The listing builds one solid part. Answer for the finished solid, in the listing's coordinates (mm). A direction names the side the tool comes from. Coordinates: 2 decimals unless noted, no trailing zeros. Order: outer loops, then holes, each group sorted by start corner. A loop starts at its lowest first (then second) coordinate and runs counter-clockwise, first axis right, second up. Notation, with made-up numbers: (42.5, 20) - (58.5, 20) arc R26 cw to (58.5, 49) - close; hole circle Ø4 at (-13, -4). An arc over 180 degrees is marked (long way). Use a Markdown table: item, result. Add a question column.
Item 1: The mould has two halves that part along X. Classify faces 1 (the flat face through (5, 38, 1)), 2 (the flat face through (-155, 38, 1)), 3 (the cylindrical face through (-43.2, -41, 130.3)): released by +X, released by -X, zero draft, split by the parting line, or undercut.
Item 2: For faces 4 (the cylindrical face through (-73.88, 1.32, 29.97)), 5 (the cylindrical face through (-149.93, 85.907, -19.077)), 6 (the flat face through (-5, 69, -69)), 7 (the flat face through (-25, -1, -137)), determine the directions among +Z, -Z, +X, -X, +Y, -Y from which every point of the face is accessible in a straight line to the end or side of a thin tool.
Item 3: Find the intervals of material crossed by line 1 along Y through (x, z) = (-34.5, 0); line 2 along X through (y, z) = (-25, -141.5); line 3 along X through (y, z) = (109.5, 16.5), in increasing order.
Item 4: The part is cut by section C-C, the plane x = -117. Give the vertices of the cut face in (y, z), then the cut area to 3 significant figures.
Item 5: Flat-ended cylindrical pins translate along their axes: P1, Ø3, axis at x = -120, y = -101.5, coming from the -Z side; P2, Ø3, axis at y = 83, z = -92.5, coming from the +X side; P3, Ø5, axis at x = -104.5, y = 104.5, coming from the -Z side. Find the tip coordinate at first contact, or state that the pin passes through.
from build123d import *

# Parameters (mm, degrees)
SKETCH1_W          = 10
SKETCH1_H          = 88
SKETCH1_W_2        = 37
SKETCH1_H_2        = 136.59637726
SKETCH2_R          = 30
CUT_EXTRUDE1_DEPTH = 500


with BuildPart() as part:
    # Sketch1 → Revolve9 (revolve)
    with BuildSketch(Plane.XY, mode=Mode.PRIVATE) as revolve9_sk:
        with Locations((-150, 44)):
            Rectangle(SKETCH1_W, SKETCH1_H)
        with BuildLine():
            Line((-145, 0), (-125, 0))
            Line((-125, 0), (-125, 136.59637726))
            Line((-125, 136.59637726), (-125, 153.19275452))
            ThreePointArc((-125, 153.19275452), (-131.59637726, 166.59637726), (-145, 160))
            Line((-145, 160), (-145, 88))
            Line((-145, 88), (-145, 0))
        make_face()
        with Locations((-106.5, 68.29818863)):
            Rectangle(SKETCH1_W_2, SKETCH1_H_2)
        Polygon((-62, 0), (-62, 136.59637726), (-75, 98.275266021), (-88, 136.59637726), (-88, 0), align=None)
        with Locations((-43.5, 68.29818863)):
            Rectangle(SKETCH1_W_2, SKETCH1_H_2)
        with BuildLine():
            Line((-5, 88), (-5, 160))
            ThreePointArc((-5, 160), (-18.40362274, 166.59637726), (-25, 153.19275452))
            Line((-25, 153.19275452), (-25, 136.59637726))
            Line((-25, 136.59637726), (-25, 0))
            Line((-25, 0), (-5, 0))
            Line((-5, 0), (-5, 88))
        make_face()
        with Locations((0, 44)):
            Rectangle(SKETCH1_W, SKETCH1_H)
    revolve(revolve9_sk.sketch.rotate(Axis((0, 0, 0), (1, 0, 0)), 90), axis=Axis((0, 0, 0), (1, 0, 0)))

    # Sketch2 → Cut-Extrude1 (cut)
    with BuildSketch(Plane(origin=(5, 0, 0), x_dir=(0, 0, -1), z_dir=(1, 0, 0))):
        Circle(SKETCH2_R)
    extrude(amount=-CUT_EXTRUDE1_DEPTH, mode=Mode.SUBTRACT)


solid = part.part
Solution:
| question | item | result |
|---|---|---|
| 1 | face 1 | released by +X |
| 1 | face 2 | released by -X |
| 1 | face 3 | undercut |
| 2 | face 4 | +X, -X |
| 2 | face 5 | -X |
| 2 | face 6 | +X |
| 2 | face 7 | none |
| 3 | line 1 | y = -136.6 to -30, 30 to 136.6 |
| 3 | line 2 | x = -145 to -125, -25 to -5 |
| 3 | line 3 | x = -145 to -79.23, -70.77 to -5 |
| 4 | outline | circle Ø273.19 at (0, 0); hole circle Ø60 at (0, 0) |
| 4 | area | 55,800 mm2 |
| 5 | P1 | stops at z = -93.05 |
| 5 | P2 | stops at x = -5 |
| 5 | P3 | stops at z = -90.85 |
